from build123d import *

# Parameters (mm, degrees)
F1_DEPTH = 6.33
F2_R     = 2
F3_R     = 3
F5_DEPTH = 8
F7_R     = 3


# Not quite as in the source:
# - a fillet or chamfer that OpenCascade refuses, or shapes differently, is made with other operations: its cross-section is extruded or revolved along the edge and cut away or added


with BuildPart() as f1:
    # F0 (on Front) → F1 (new body)
    with BuildSketch(Plane.XZ):
        Polygon((34, 4), (-30, 14.5), (-30.2323504967, 12), (24, 2.9564342819), (24, -2.9564342819), (-30.2323504967, -12), (-30, -14.5), (34, -4), align=None)
    extrude(amount=F1_DEPTH)

    # F2
    f2_edges = [f1.edges().sort_by_distance(p)[0] for p in [
        (24, -3.165, -2.956434),
        (24, -3.165, 2.956434),
    ]]
    fillet(f2_edges, radius=F2_R)

    # F3
    f3_edges = [f1.edges().sort_by_distance(p)[0] for p in [
        (34, -3.165, 4),
        (34, -3.165, -4),
    ]]
    fillet(f3_edges, radius=F3_R)

    # F4 (on face) → F5 (join)
    with BuildSketch(Plane(origin=(1.5302228826, 0, 9.3270728083), x_dir=(0.9868074809, 0, -0.1618981023), z_dir=(0.1618981023, 0, 0.9868074809))):
        with BuildLine():
            ThreePointArc((-28.7867469125, -6.33), (-26.54875395, -5.4029929625), (-25.6217469125, -3.165))
            ThreePointArc((-25.6217469125, -3.165), (-26.54875395, -0.9270070375), (-28.7867469125, 0))
            ThreePointArc((-28.7867469125, 0), (-31.0247398749, -0.9270070375), (-31.9517469125, -3.165))
            ThreePointArc((-31.9517469125, -3.165), (-31.0247398749, -5.4029929625), (-28.7867469125, -6.33))
        make_face()
    extrude(amount=F5_DEPTH)

    # F6: fillet of radius 2 on 1 edges, made by hand

    # F6_s1 → F6_t2 (revolve, cut)
    with BuildSketch(Plane.XZ.offset(3.165)):
        with BuildLine():
            ThreePointArc((-29.0286113859, 20.4208448857), (-28.221594455, 21.7215636961), (-26.7312002194, 22.0706636429))
            Line((-26.7312002194, 22.0706636429), (-28.7048151813, 22.3944598476))
            Line((-28.7048151813, 22.3944598476), (-29.0286113859, 20.4208448857))
        make_face()
    revolve(axis=Axis((-25.581569504, -3.165, 21.8820523537), (-0.1618981023, 0, -0.9868074809)), mode=Mode.SUBTRACT)

    # F7
    f7_edges = [f1.edges().sort_by_distance(p)[0] for p in [
        (-30.116175, 0, 13.25),
        (-30.116175, -6.33, 13.25),
        (-30.116175, 0, -13.25),
        (-30.116175, -6.33, -13.25),
    ]]
    fillet(f7_edges, radius=F7_R)


solid = f1.part
Read the model definition and answer for the solid it produces. Units are mm, in the model's axes. A direction names the side the tool comes from. Coordinates: 2 decimals unless noted, no trailing zeros. Write each loop counter-clockwise with the first axis right and the second up, starting at its lowest first coordinate (ties: lowest second). Pieces come first, ordered by that corner, then holes. Notation, with made-up numbers: (-8.5, -7) - (19.5, -7) arc R22 ccw to (19.5, 30) - close; hole circle Ø6 at (-38, 59). An arc over 180 degrees is marked (long way). One line per question, with ' | ' between items.
Q1. Find section A-A, the plane x = -2. Write down the section's boundary in (y, z).
Result set:
outline: (-6.33, -9.91) - (0, -9.91) - (0, -7.29) - (-6.33, -7.29) - close; (-6.33, 7.29) - (0, 7.29) - (0, 9.91) - (-6.33, 9.91) - close
Q2. Consider L1, parallel to X at y = -6, z = -0.5; L2, parallel to Z at x = 1.5, y = -1.75; L3, parallel to Z at x = 23, y = -5.75. Determine where each line is inside the solid, lowest interval first. Write a range as [from, to].
Result set:
L1: [24, 34] | L2: [-9.33, -6.71], [6.71, 9.33] | L3: [-5.8, -2.99], [2.99, 5.8]
Q3. For faces 1 (the cylindrical face through (23.513, -3.209, 2.57)), 2 (the cylindrical face through (33.306, -3.209, -3.371)), determine the directions among +Z, -Z, +X, -X, +Y, -Y from which every point of the face is accessible in a straight line to the end or side of a thin tool.
Result set:
face 1: -X, +Y, -Y | face 2: -Z, +X, +Y, -Y
Q4. Find section B-B, the plane x = -16. Write down the section's boundary in (y, z), plus the area to 3 significant figures.
Result set:
outline: (-6.33, -12.2) - (0, -12.2) - (0, -9.63) - (-6.33, -9.63) - close; (-6.33, 9.63) - (0, 9.63) - (0, 12.2) - (-6.33, 12.2) - close | area: 32.6 mm^2
Q5. Find section D-D, the plane z = -7. Write down the section's boundary in (x, y).
Result set:
outline: (-0.25, -6.33) - (15.71, -6.33) - (15.71, 0) - (-0.25, 0) - close
Q6. Each of these flat-tipped pins is pushed along its axis until it touches: P1, Ø1, axis at y = -4, z = 4.5, coming from the +X side; P2, Ø1.3, axis at y = -2.5, z = -0.5, coming from the -X side. Where does it stop, or does it pass through?
Result set:
P1: x = 32.58 | P2: x = 24
Q7. Find section C-C, the plane z = 0. Write down the section's boundary in (x, y), plus the area to 3 significant figures.
Result set:
outline: (24, -6.33) - (34, -6.33) - (34, 0) - (24, 0) - close | area: 63.3 mm^2
